For this review, take the finished solid that the model builds, in its own axes (mm). A direction names the side the tool comes from. Coordinates: 2 decimals unless noted, no trailing zeros. Loops run counter-clockwise (first coordinate to the right, second up) from the corner with the lowest first, then second, coordinate; pieces in that order, holes last. Notation, with made-up numbers: (-26.75, 0.5) -> (10.25, 0.5) arc R21 ccw to (10.25, 14.5) -> close; hole circle Ø2 at (37.25, 72.25). An arc over 180 degrees is marked (long way). Answer in a Markdown table with one row per item.
from build123d import *

# Parameters (mm, degrees)
SKETCH1_W               = 36.068
SKETCH1_H               = 38.1
BOSS_EXTRUDE1_DEPTH     = 63.5
SKETCH3_W               = 36.068
SKETCH3_H               = 10.16
CUT_EXTRUDE1_DEPTH      = 38.1
SKETCH4_W               = 36.068
SKETCH4_H               = 17.145
CUT_EXTRUDE2_DEPTH      = 19.05
SKETCH5_W               = 17.399
SKETCH5_H               = 10.16
CUT_EXTRUDE3_DEPTH      = 47.257298408
CUT_EXTRUDE4_DEPTH      = 71.283227416
CUT_EXTRUDE4_DEPTH_BACK = 71.283227416
SKETCH6_R               = 1.125
SKETCH7_W               = 13.589
SKETCH7_H               = 38.1
CUT_EXTRUDE6_DEPTH      = 69.705004592
SKETCH8_W               = 10.16
SKETCH8_H               = 6.35
BOSS_EXTRUDE2_DEPTH     = 3.81


with BuildPart() as part:
    # Sketch1 → Boss-Extrude1 (new body)
    with BuildSketch(Plane(origin=(0, 0, 0), x_dir=(1, 0, 0), z_dir=(0, 1, 0))):
        Rectangle(SKETCH1_W, SKETCH1_H)
    extrude(amount=BOSS_EXTRUDE1_DEPTH)

    # Sketch3 → Cut-Extrude1 (cut)
    with BuildSketch(Plane(origin=(0, 63.5, 0), x_dir=(1, 0, 0), z_dir=(0, 1, 0))):
        Rectangle(SKETCH3_W, SKETCH3_H)
    extrude(amount=-CUT_EXTRUDE1_DEPTH, mode=Mode.SUBTRACT)

    # Sketch4 → Cut-Extrude2 (cut)
    with BuildSketch(Plane.XZ):
        Rectangle(SKETCH4_W, SKETCH4_H)
    extrude(amount=-CUT_EXTRUDE2_DEPTH, mode=Mode.SUBTRACT)

    # Sketch5 → Cut-Extrude3 (cut, through all)
    with BuildSketch(Plane(origin=(0, 25.4, 0), x_dir=(1, 0, 0), z_dir=(0, 1, 0))):
        with Locations((-9.3345, 0)):
            Rectangle(SKETCH5_W, SKETCH5_H)
        with Locations((9.3345, 0)):
            Rectangle(SKETCH5_W, SKETCH5_H)
    extrude(amount=-CUT_EXTRUDE3_DEPTH, mode=Mode.SUBTRACT)

    # Sketch6 → Cut-Extrude4 (cut, two sides: drawn at the far end of the back side and taken through both)
    with BuildSketch(Plane.XY.offset(-5.08).offset(-CUT_EXTRUDE4_DEPTH_BACK)):
        with Locations((0, 29.845)):
            Circle(SKETCH6_R)
    extrude(amount=CUT_EXTRUDE4_DEPTH + CUT_EXTRUDE4_DEPTH_BACK, mode=Mode.SUBTRACT)

    # Sketch7 → Cut-Extrude6 (cut, through all)
    with BuildSketch(Plane(origin=(0, 63.5, 0), x_dir=(1, 0, 0), z_dir=(0, 1, 0))):
        with Locations((11.2395, 0)):
            Rectangle(SKETCH7_W, SKETCH7_H)
    extrude(amount=-CUT_EXTRUDE6_DEPTH, mode=Mode.SUBTRACT)

    # Sketch8 → Boss-Extrude2 (add)
    with BuildSketch(Plane(origin=(0.635, 0, 0), x_dir=(0, 0, -1), z_dir=(1, 0, 0))):
        with Locations((0, 22.225)):
            Rectangle(SKETCH8_W, SKETCH8_H)
    extrude(amount=BOSS_EXTRUDE2_DEPTH)


solid = part.part
Item 1: For L1, parallel to Z at x = 3.25, y = 38.5; L2, parallel to Y at x = 0, z = -13.25; L3, parallel to Z at x = -10.75, y = 17, list the stretches that pass through material, from the lowest coordinate up.
Worked answers:
| item | result |
|---|---|
| L1 | -19.05 to -5.08, 5.08 to 19.05 |
| L2 | 0 to 28.72, 30.97 to 63.5 |
| L3 | -19.05 to -8.57, 8.57 to 19.05 |
Item 2: Insertion check: pin 1 (5 mm diameter, centred on y = 20.5, z = 1.5, fed in from -X) (3 decimals); pin 2 (1.3 mm diameter, centred on x = 0, y = 29.845, fed in from -Z); pin 3 (2.5 mm diameter, centred on x = 2.5, z = 2, fed in from +Y). Each pin has a flat end and moves straight along its axis. Give the tip position at first contact, or say it passes through.
Worked answers:
| item | result |
|---|---|
| pin 1 | x = -0.635 |
| pin 2 | through |
| pin 3 | y = 25.4 |
Item 3: Take a section at B-B, the plane x = -14.5. State the section outline as (y, z) points, and give its area (3 significant figures).
Worked answers:
| item | result |
|---|---|
| outline | (0, -19.05) -> (63.5, -19.05) -> (63.5, -5.08) -> (19.05, -5.08) -> (19.05, -8.57) -> (0, -8.57) -> close; (0, 8.57) -> (19.05, 8.57) -> (19.05, 5.08) -> (63.5, 5.08) -> (63.5, 19.05) -> (0, 19.05) -> close |
| area | 1,640 mm² |
Item 4: Take a section at A-A, the plane x = 0. State the section outline as (y, z) points.
Worked answers:
| item | result |
|---|---|
| outline | (0, -19.05) -> (28.72, -19.05) -> (28.72, -5.08) -> (25.4, -5.08) -> (25.4, 5.08) -> (28.72, 5.08) -> (28.72, 19.05) -> (0, 19.05) -> (0, 8.57) -> (19.05, 8.57) -> (19.05, -8.57) -> (0, -8.57) -> close; (30.97, -19.05) -> (63.5, -19.05) -> (63.5, -5.08) -> (30.97, -5.08) -> close; (30.97, 5.08) -> (63.5, 5.08) -> (63.5, 19.05) -> (30.97, 19.05) -> close |
Item 5: Take a section at C-C, the plane y = 38. State the section outline as (x, z) points (3 decimals).
Worked answers:
| item | result |
|---|---|
| outline | (-18.034, -19.05) -> (4.445, -19.05) -> (4.445, -5.08) -> (-18.034, -5.08) -> close; (-18.034, 5.08) -> (4.445, 5.08) -> (4.445, 19.05) -> (-18.034, 19.05) -> close |
Item 6: For faces 1 (the flat face through (2, 25.4, 0)), 2 (the flat face through (1, 19.05, 0)), 3 (the flat face through (-18.034, 31, 12)), list the 3-axis set-ups (+Z, -Z, +X, -X, +Y, -Y) from which the entire face can be reached by the end or side of a thin tool; tool diameter is ignored.
Worked answers:
| item | result |
|---|---|
| face 1 | +X, -X, +Y |
| face 2 | +X, -X, -Y |
| face 3 | +Z, -Z, -X, +Y, -Y |
Item 7: The part is to be moulded in two halves that separate along Z. For faces 4 (the flat face through (-7, 31, -19.05)), 5 (the cylindrical face through (-0.15, 30.96, -12.16)), 6 (the flat face through (-0.635, 22, 0)), 7 (the flat face through (-7, 9, 8.572)), say which applies: +Z half, -Z half, draft (parallel to the pull), parting line (faces both ways), or undercut.
Worked answers:
| item | result |
|---|---|
| face 4 | -Z half |
| face 5 | draft |
| face 6 | undercut |
| face 7 | undercut |
Item 8: Take a section at D-D, the plane y = 24.5. State the section outline as (x, z) points (3 decimals).
Worked answers:
| item | result |
|---|---|
| outline | (-18.034, -19.05) -> (4.445, -19.05) -> (4.445, 19.05) -> (-18.034, 19.05) -> (-18.034, 5.08) -> (-0.635, 5.08) -> (-0.635, -5.08) -> (-18.034, -5.08) -> close |
